```python
from build123d import *

# Parameters (mm, degrees)
SKETCH_W           = 100
SKETCH_H           = 100
PAD_DEPTH          = 12
SKETCH001_W        = 40
SKETCH001_H        = 40
PAD001_DEPTH       = 48
PAD002_DEPTH       = 5
POLARPATTERN_COUNT = 4


with BuildPart() as part:
    # Sketch → Pad (new body)
    with BuildSketch(Plane.XY):
        Rectangle(SKETCH_W, SKETCH_H)
    extrude(amount=PAD_DEPTH)

    # Sketch001 (on Face6 of Pad) → Pad001 (join)
    with BuildSketch(Plane.XY.offset(12)):
        Rectangle(SKETCH001_W, SKETCH001_H)
    extrude(amount=PAD001_DEPTH)

    # Sketch002 → Pad002 (join, symmetric)
    with BuildSketch(Plane.XZ):
        Polygon((20, 60), (20, 12), (50, 12), align=None)
    pad002 = extrude(amount=PAD002_DEPTH, both=True)

    # PolarPattern: Pad002 ×4 about axis
    polarpattern_axis = Axis((0, 0, 0), (0, 0, 1))
    for i in range(1, POLARPATTERN_COUNT):
        add(pad002.rotate(polarpattern_axis, i * 360 / POLARPATTERN_COUNT))


solid = part.part
```
Source: CAD feature listing. Evaluate the final solid. Frame: model axes, mm. A direction names the side the tool comes from. Coordinates: 2 decimals unless noted, no trailing zeros. Loops run counter-clockwise (first coordinate to the right, second up) from the corner with the lowest first, then second, coordinate; pieces in that order, holes last. Notation, with made-up numbers: M 70.5,-34.5 L 109.5,-34.5 A18 cw 109.5,-19.5 Z; hole C 26,63 d4. An arc over 180 degrees is marked long. Put each result on its own line as item: value. Start each with the question number.
1) Cut plane A-A on z = 54. Return the cut outline in (x, y).
2) Cut plane D-D on z = 48. Return the cut outline in (x, y), then the cut area to 3 significant figures.
3) Reachability of faces 1 (the face through (-5, -28, 26)), 2 (the face through (28, 5, 26)), 3 (the face through (-5, 28, 26)) from +Z, -Z, +X, -X, +Y, -Y: full face, straight path, thin tool, end or side. Return the list, or none.
4) Ray query, L1, parallel to Z at x = -18.5, y = 22; L2, parallel to Y at x = -18.5, z = 48; L3, parallel to X at y = 26, z = 28.5. Return the intervals inside material, ascending. Write a range as from..to.
5) Cut plane B-B on y = 39.5. Return the cut outline in (x, z).
6) Contact query for flat-ended pins moving along their axis: pin 1 Ø2 at (x, z) = (-36, 17) entering from +Y; pin 2 Ø15 at (y, z) = (-31.5, 30) entering from -X; pin 3 Ø12 at (x, z) = (28.5, 28) entering from -Y. Output: stop coordinate, or through.
7) Cut plane C-C on x = 1.5. Return the cut outline in (y, z), then the cut area to 3 significant figures.
The answers:
1. outline: M -23.75,-5 L -20,-5 L -20,-20 L -5,-20 L -5,-23.75 L 5,-23.75 L 5,-20 L 20,-20 L 20,-5 L 23.75,-5 L 23.75,5 L 20,5 L 20,20 L 5,20 L 5,23.75 L -5,23.75 L -5,20 L -20,20 L -20,5 L -23.75,5 Z
2. outline: M -27.5,-5 L -20,-5 L -20,-20 L -5,-20 L -5,-27.5 L 5,-27.5 L 5,-20 L 20,-20 L 20,-5 L 27.5,-5 L 27.5,5 L 20,5 L 20,20 L 5,20 L 5,27.5 L -5,27.5 L -5,20 L -20,20 L -20,5 L -27.5,5 Z
2. area: 1,900 mm²
3. face 1: +Z, -X, -Y
3. face 2: +Z, +X, +Y
3. face 3: +Z, -X, +Y
4. L1: z = 0..12
4. L2: y = -20..20
4. L3: x = -5..5
5. outline: M -50,0 L 50,0 L 50,12 L 5,12 L 5,28.8 L -5,28.8 L -5,12 L -50,12 Z
6. pin 1: stops at y = 5
6. pin 2: stops at x = -5
6. pin 3: stops at y = -5
7. outline: M -50,0 L 50,0 L 50,12 L 20,60 L -20,60 L -50,12 Z
7. area: 4,560 mm²
